Check sheet for the modelled part. Datum: model origin and axes. Units: mm. A direction names the side the tool comes from. Give positions to 0.01 mm unless a question says otherwise; leave off trailing zeros. Write each loop counter-clockwise with the first axis right and the second up, starting at its lowest first coordinate (ties: lowest second). Pieces come first, ordered by that corner, then holes. Notation, with made-up numbers: (65.5, 64.25) -> (108.5, 64.25) arc R16 ccw to (108.5, 73.25) -> close; hole circle Ø5 at (-27.5, 35). An arc over 180 degrees is marked (long way). Return JSON: item names as keys, results as strings.
from build123d import *

# Parameters (mm, degrees)
SKETCH1_R           = 1
SKETCH1_R_2         = 6.35
SKETCH1_R_3         = 4
SKETCH1_R_4         = 3.5
SKETCH1_R_5         = 1.65
BOSS_EXTRUDE3_DEPTH = 6.3


with BuildPart() as part:
    # Sketch1 → Boss-Extrude3 (new body)
    with BuildSketch(Plane(origin=(0, 0, 0), x_dir=(1, 0, 0), z_dir=(0, 1, 0))):
        with BuildLine():
            Line((0, -65), (0, 65))
            ThreePointArc((0, 65), (6.670628594, 73.693332437), (16.794228634, 69.5))
            Line((16.794228634, 69.5), (34.692086979, 38.5))
            ThreePointArc((34.692086979, 38.5), (37.986315613, 35.205771366), (42.486315613, 34))
            Line((42.486315613, 34), (101.527767497, 34))
            ThreePointArc((101.527767497, 34), (107.891728528, 31.363961031), (110.527767497, 25))
            Line((110.527767497, 25), (110.527767497, -25))
            ThreePointArc((110.527767497, -25), (107.891728528, -31.363961031), (101.527767497, -34))
            Line((101.527767497, -34), (42.486315613, -34))
            ThreePointArc((42.486315613, -34), (37.986315613, -35.205771366), (34.692086979, -38.5))
            Line((34.692086979, -38.5), (16.794228634, -69.5))
            ThreePointArc((16.794228634, -69.5), (6.670628594, -73.693332437), (0, -65))
        make_face()
        with Locations(Location((9, 65, 0), (0, 0, 270))):
            Circle(SKETCH1_R, mode=Mode.SUBTRACT)
        with Locations(Location((46.527767497, 0, 0), (0, 0, 90))):
            Circle(SKETCH1_R_2, mode=Mode.SUBTRACT)
        with Locations(Location((101.527767497, 0, 0), (0, 0, 90))):
            Circle(SKETCH1_R_3, mode=Mode.SUBTRACT)
        with Locations(Location((20, 25.4, 0), (0, 0, 270))):
            Circle(SKETCH1_R_4, mode=Mode.SUBTRACT)
        with Locations(Location((45.4, 25.4, 0), (0, 0, 270))):
            Circle(SKETCH1_R_4, mode=Mode.SUBTRACT)
        with Locations(Location((45.4, -25.4, 0), (0, 0, 90))):
            Circle(SKETCH1_R_4, mode=Mode.SUBTRACT)
        with Locations(Location((20, -25.4, 0), (0, 0, 90))):
            Circle(SKETCH1_R_4, mode=Mode.SUBTRACT)
        with Locations(Location((9, -65, 0), (0, 0, 90))):
            Circle(SKETCH1_R, mode=Mode.SUBTRACT)
        with Locations(Location((89.027767497, -25, 0), (0, 0, 270))):
            Circle(SKETCH1_R_5, mode=Mode.SUBTRACT)
        with Locations(Location((65.027767497, -25, 0), (0, 0, 270))):
            Circle(SKETCH1_R_5, mode=Mode.SUBTRACT)
        with Locations(Location((65.027767497, 25, 0), (0, 0, 90))):
            Circle(SKETCH1_R_5, mode=Mode.SUBTRACT)
        with Locations(Location((89.027767497, 25, 0), (0, 0, 90))):
            Circle(SKETCH1_R_5, mode=Mode.SUBTRACT)
    extrude(amount=BOSS_EXTRUDE3_DEPTH)


solid = part.part
(1) Cross-section at B-B on y = 1. State how many separate pieces and enclosed holes the cut face has, then the cut area to 3 significant figures.
Reply:
{"separate pieces": "1", "enclosed holes": "12", "area": "9,130 mm^2"}
(2) Cross-section at D-D on z = -47. Enter the section's corners in (x, y).
Reply:
{"outline": "(0, 0) -> (29.78, 0) -> (29.78, 6.3) -> (0, 6.3) -> close"}
(3) Cross-section at C-C on x = 70. Enter the section's corners in (y, z).
Reply:
{"outline": "(0, -34) -> (6.3, -34) -> (6.3, 34) -> (0, 34) -> close"}
(4) Thickness scan on L1, parallel to X at y = 1.5, z = -25; L2, parallel to X at y = 2, z = 0; L3, parallel to Z at x = 48, y = 3.75. Record the ranges inside material, lowest first.
Reply:
{"L1": "0 to 16.52, 23.48 to 41.92, 48.88 to 63.38, 66.68 to 87.38, 90.68 to 110.53", "L2": "0 to 40.18, 52.88 to 97.53, 105.53 to 110.53", "L3": "-34 to -27.74, -23.06 to -6.18, 6.18 to 23.06, 27.74 to 34"}
(5) Set-up check for faces 1 (the flat face through (72, 3, -34)), 2 (the cylindrical face through (65.1, 3.11, 23.35)): record each of +Z, -Z, +X, -X, +Y, -Y from which the full face is reachable in a straight line by a thin tool's end or side.
Reply:
{"face 1": "-Z, +X, +Y, -Y", "face 2": "+Y, -Y"}
(6) Cross-section at A-A on z = 0. Enter the section's corners in (x, y), then the cut area to 3 significant figures.
Reply:
{"outline": "(0, 0) -> (40.18, 0) -> (40.18, 6.3) -> (0, 6.3) -> close; (52.88, 0) -> (97.53, 0) -> (97.53, 6.3) -> (52.88, 6.3) -> close; (105.53, 0) -> (110.53, 0) -> (110.53, 6.3) -> (105.53, 6.3) -> close", "area": "566 mm^2"}
(7) Release check for a two-part mould opening along Z. For faces 3 (the cylindrical face through (17.05, 3.11, 23.52)), 4 (the flat face through (25.87, 3.11, 53.78)), 5 (the flat face through (110.528, 3, 0)) record: pulls with the +Z half, pulls with the -Z half, needs draft (parallel to the pull), parting line crosses it, or undercut.
Reply:
{"face 3": "undercut", "face 4": "pulls with the +Z half", "face 5": "needs draft"}
